Design review of the part built by this model. Coordinates are the model's own, in mm. Round coordinates to 2 decimals unless told otherwise and drop trailing zeros. Loops run counter-clockwise (first coordinate to the right, second up) from the corner with the lowest first, then second, coordinate; pieces in that order, holes last. Notation, with made-up numbers: (72.5, -35) - (79.5, -35) arc R23 cw to (79.5, -8) - close; hole circle Ø7 at (65.25, 65.25). An arc over 180 degrees is marked (long way). Return JSON: item names as keys, results as strings. Group by question number.
(1) We need section C-C, the plane x = -13. Write out the cut boundary in (y, z).
(2) We need section A-A, the plane y = 1.75. Write out the cut boundary in (x, z).
(3) Wall thickness on L1, parallel to Z at x = -2, y = 1.35; L2, parallel to X at y = 1.1, z = 1.5; L3, parallel to X at y = 1.7, z = 30.5: over which ranges is each line inside the solid? List them lowest first. Write a range as [from, to].
(4) We need section B-B, the plane z = -54.5. Write out the cut boundary in (x, y).
(5) Clearance check with flat-ended pins moving along their axes: pin 1 (2 mm diameter, centred on x = 94.5, y = 2.5, fed in from -Z); pin 2 (2 mm diameter, centred on y = 1, z = -62, fed in from -X); pin 3 (1.2 mm diameter, centred on y = 1.5, z = -38, fed in from +X). State where each tip first meets the part, or that it passes through.
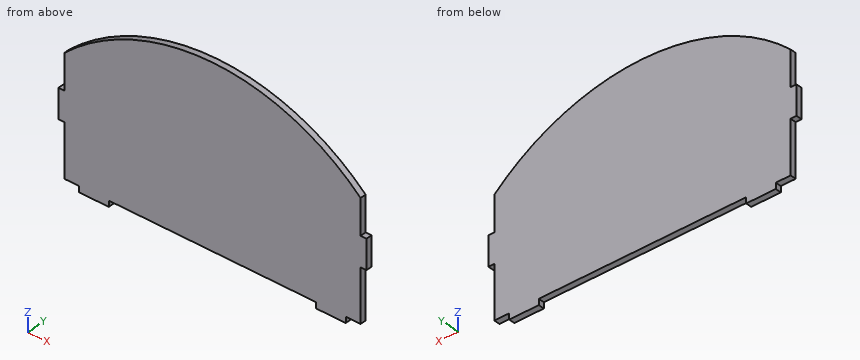
from build123d import *

# Parameters (mm, degrees)
EXTRUDE1_DEPTH = 4


with BuildPart() as part:
    # Sketch1 → Extrude1 (new body)
    with BuildSketch(Plane(origin=(0, 0, 0), x_dir=(1, 0, 0), z_dir=(0, 1, 0))):
        with BuildLine():
            Line((-90, 60), (-100, 60))
            Line((-100, 60), (-100, 24))
            Line((-100, 24), (-104, 24))
            Line((-104, 24), (-104, 4))
            Line((-104, 4), (-100, 4))
            Line((-100, 4), (-100, -20))
            ThreePointArc((-100, -20), (0, -60), (100, -20))
            Line((100, -20), (100, 4))
            Line((100, 4), (104, 4))
            Line((104, 4), (104, 24))
            Line((104, 24), (100, 24))
            Line((100, 24), (100, 60))
            Line((100, 60), (90, 60))
            Line((90, 60), (90, 64))
            Line((90, 64), (70, 64))
            Line((70, 64), (70, 60))
            Line((70, 60), (-70, 60))
            Line((-70, 60), (-70, 64))
            Line((-70, 64), (-90, 64))
            Line((-90, 64), (-90, 60))
        make_face()
    extrude(amount=EXTRUDE1_DEPTH)


solid = part.part
Solutions:
{
 "1": {"outline": "(0, -60) - (4, -60) - (4, 59.42) - (0, 59.42) - close"},
 "2": {"outline": "(-104, -24) - (-100, -24) - (-100, -60) - (-90, -60) - (-90, -64) - (-70, -64) - (-70, -60) - (70, -60) - (70, -64) - (90, -64) - (90, -60) - (100, -60) - (100, -24) - (104, -24) - (104, -4) - (100, -4) - (100, 20) arc R145 ccw to (-100, 20) - (-100, -4) - (-104, -4) - close"},
 "3": {"L1": "[-60, 59.99]", "L2": "[-100, 100]", "L3": "[-87.66, 87.66]"},
 "4": {"outline": "(-100, 0) - (100, 0) - (100, 4) - (-100, 4) - close"},
 "5": {"pin 1": "z = -60", "pin 2": "x = -90", "pin 3": "x = 100"}
}
